Build history of the part. All positions in model axes, mm. Round coordinates to 2 decimals unless told otherwise and drop trailing zeros. Write each loop counter-clockwise with the first axis right and the second up, starting at its lowest first coordinate (ties: lowest second). Pieces come first, ordered by that corner, then holes. Notation, with made-up numbers: (-37, -20) -> (-3, -20) arc R31 cw to (-3, 19) -> close; hole circle Ø9 at (-1, -11.5). An arc over 180 degrees is marked (long way). Return JSON: item names as keys, results as strings.
from build123d import *

# Parameters (mm, degrees)
SKETCH2_W           = 7
SKETCH2_H           = 10.3
SKETCH2_H_2         = 2.08
BOSS_EXTRUDE1_DEPTH = 0.1


with BuildPart() as part:
    # Sketch2 → Boss-Extrude1 (new body)
    with BuildSketch(Plane(origin=(0, 0, 0), x_dir=(1, 0, 0), z_dir=(0, 1, 0))):
        with BuildLine():
            Line((-0.6, 9.5), (-1.75, 9.5))
            ThreePointArc((-1.75, 9.5), (-4.048097039, 8.548097039), (-5, 6.25))
            Line((-5, 6.25), (-5, -6.25))
            ThreePointArc((-5, -6.25), (-4.048097039, -8.548097039), (-1.75, -9.5))
            Line((-1.75, -9.5), (-0.6, -9.5))
            Line((-0.6, -9.5), (-0.6, -8.65))
            ThreePointArc((-0.6, -8.65), (0, -8.05), (0.6, -8.65))
            Line((0.6, -8.65), (0.6, -9.5))
            Line((0.6, -9.5), (1.75, -9.5))
            ThreePointArc((1.75, -9.5), (4.048097039, -8.548097039), (5, -6.25))
            Line((5, -6.25), (5, 6.25))
            ThreePointArc((5, 6.25), (4.048097039, 8.548097039), (1.75, 9.5))
            Line((1.75, 9.5), (0.6, 9.5))
            Line((0.6, 9.5), (0.6, 8.65))
            ThreePointArc((0.6, 8.65), (0, 8.05), (-0.6, 8.65))
            Line((-0.6, 8.65), (-0.6, 9.5))
        make_face()
        with Locations((0, 2.15)):
            Rectangle(SKETCH2_W, SKETCH2_H, mode=Mode.SUBTRACT)
        with Locations((0, -6.26)):
            Rectangle(SKETCH2_W, SKETCH2_H_2, mode=Mode.SUBTRACT)
    extrude(amount=BOSS_EXTRUDE1_DEPTH)


solid = part.part
Q1. Wall check: L1, parallel to Z at x = 1.25, y = 0.05; L2, parallel to X at y = 0.05, z = 0.75; L3, parallel to Z at x = -3, y = 0.05. Give the ranges that are in metal, low to high.
Verdict:
{"L1": "z = -9.5 to -7.3, 3 to 5.22, 7.3 to 9.5", "L2": "x = -5 to -3.5, 3.5 to 5", "L3": "z = -9.25 to -7.3, 3 to 5.22, 7.3 to 9.25"}
Q2. Saw through at D-D on z = -6.5. List the corners of the cut face in (x, y).
Verdict:
{"outline": "(-4.99, 0) -> (-3.5, 0) -> (-3.5, 0.1) -> (-4.99, 0.1) -> close; (3.5, 0) -> (4.99, 0) -> (4.99, 0.1) -> (3.5, 0.1) -> close"}
Q3. Saw through at A-A on z = -1.25. List the corners of the cut face in (x, y).
Verdict:
{"outline": "(-5, 0) -> (-3.5, 0) -> (-3.5, 0.1) -> (-5, 0.1) -> close; (3.5, 0) -> (5, 0) -> (5, 0.1) -> (3.5, 0.1) -> close"}
Q4. Saw through at B-B on x = 0. List the corners of the cut face in (y, z).
Verdict:
{"outline": "(0, -8.05) -> (0.1, -8.05) -> (0.1, -7.3) -> (0, -7.3) -> close; (0, 3) -> (0.1, 3) -> (0.1, 5.22) -> (0, 5.22) -> close; (0, 7.3) -> (0.1, 7.3) -> (0.1, 8.05) -> (0, 8.05) -> close"}
